Check sheet for the modelled part. Datum: model origin and axes. Units: mm. Face numbers are marked on the shaded views. A direction names the side the tool comes from. Coordinates: 2 decimals unless noted, no trailing zeros. Write each loop counter-clockwise with the first axis right and the second up, starting at its lowest first coordinate (ties: lowest second). Pieces come first, ordered by that corner, then holes. Notation, with made-up numbers: (84.5, 40.5) -> (114.5, 40.5) arc R22 cw to (114.5, 50.5) -> close; hole circle Ø1 at (-25.5, 51). An arc over 180 degrees is marked (long way). One line per item, written item: value. Start each with the question number.
1) Scan lines: line 1 along Y through (x, z) = (0, -3.25); line 2 along Y through (x, z) = (12, -1.5); line 3 along Z through (x, y) = (-11, -18.5). Record each from-to range of solid material in increasing order. Write a range as [from, to].
2) Set-up check for the marked faces 1, 2 and 3: record each of +Z, -Z, +X, -X, +Y, -Y from which the full face is reachable in a straight line by a thin tool's end or side.
3) Gauge pin test, flat ends, axial feed: P1, Ø1.6, axis at x = 12.5, y = 0, coming from the -Z side; P2, Ø3, axis at y = -8.5, z = 20.5, coming from the +X side (3 decimals); P3, Ø8, axis at y = -6.5, z = 30, coming from the -X side. Record the tip position at first contact, or that the pin passes through.
4) Sectioned sample at D-D on z = 18.5. Enter the section's corners in (x, y).
5) Sectioned sample at C-C on z = -1. Enter the section's corners in (x, y).
6) Sectioned sample at A-A on y = 0. Enter the section's corners in (x, z), plus the area to 3 significant figures.
```python
from build123d import *

# Parameters (mm, degrees)
SKETCH1_R           = 24
SKETCH1_R_2         = 1
BOSS_EXTRUDE1_DEPTH = 9.4
SKETCH1_4_R         = 20
SKETCH1_4_R_2       = 17.5
SKETCH1_4_R_3       = 1
BOSS_EXTRUDE2_DEPTH = 37
SKETCH1_5_R         = 17.5
SKETCH1_5_R_2       = 1
BOSS_EXTRUDE3_DEPTH = 4.5


with BuildPart() as part:
    # Sketch1 → Boss-Extrude1 (new body)
    with BuildSketch(Plane.XY):
        Circle(SKETCH1_R)
        with Locations((0, 12.5)):
            Circle(SKETCH1_R_2, mode=Mode.SUBTRACT)
        with Locations((12.5, 0)):
            Circle(SKETCH1_R_2, mode=Mode.SUBTRACT)
        with Locations((0, -12.5)):
            Circle(SKETCH1_R_2, mode=Mode.SUBTRACT)
        with Locations((-12.5, 0)):
            Circle(SKETCH1_R_2, mode=Mode.SUBTRACT)
    extrude(amount=BOSS_EXTRUDE1_DEPTH)

    # Sketch1_4 → Boss-Extrude2 (add)
    # profile 1 of 6: a face of its own
    with BuildSketch(Plane.XY):
        Circle(SKETCH1_4_R)
        Circle(SKETCH1_4_R_2, mode=Mode.SUBTRACT)
    # profile 2 of 6: a face of its own
    with BuildSketch(Plane.XY):
        Circle(SKETCH1_4_R_2)
        with Locations((-12.5, 0)):
            Circle(SKETCH1_4_R_3, mode=Mode.SUBTRACT)
        with Locations((0, -12.5)):
            Circle(SKETCH1_4_R_3, mode=Mode.SUBTRACT)
        with Locations((12.5, 0)):
            Circle(SKETCH1_4_R_3, mode=Mode.SUBTRACT)
        with Locations((0, 12.5)):
            Circle(SKETCH1_4_R_3, mode=Mode.SUBTRACT)
    # profile 3 of 6: a face of its own
    with BuildSketch(Plane.XY):
        with Locations((0, 12.5)):
            Circle(SKETCH1_4_R_3)
    # profile 4 of 6: a face of its own
    with BuildSketch(Plane.XY):
        with Locations((-12.5, 0)):
            Circle(SKETCH1_4_R_3)
    # profile 5 of 6: a face of its own
    with BuildSketch(Plane.XY):
        with Locations((12.5, 0)):
            Circle(SKETCH1_4_R_3)
    # profile 6 of 6: a face of its own
    with BuildSketch(Plane.XY):
        with Locations((0, -12.5)):
            Circle(SKETCH1_4_R_3)
    extrude(amount=BOSS_EXTRUDE2_DEPTH)

    # Sketch1_5 → Boss-Extrude3 (add)
    with BuildSketch(Plane.XY):
        Circle(SKETCH1_5_R)
        with Locations((0, 12.5)):
            Circle(SKETCH1_5_R_2, mode=Mode.SUBTRACT)
        with Locations((12.5, 0)):
            Circle(SKETCH1_5_R_2, mode=Mode.SUBTRACT)
        with Locations((0, -12.5)):
            Circle(SKETCH1_5_R_2, mode=Mode.SUBTRACT)
        with Locations((-12.5, 0)):
            Circle(SKETCH1_5_R_2, mode=Mode.SUBTRACT)
    extrude(amount=-BOSS_EXTRUDE3_DEPTH)


solid = part.part
```
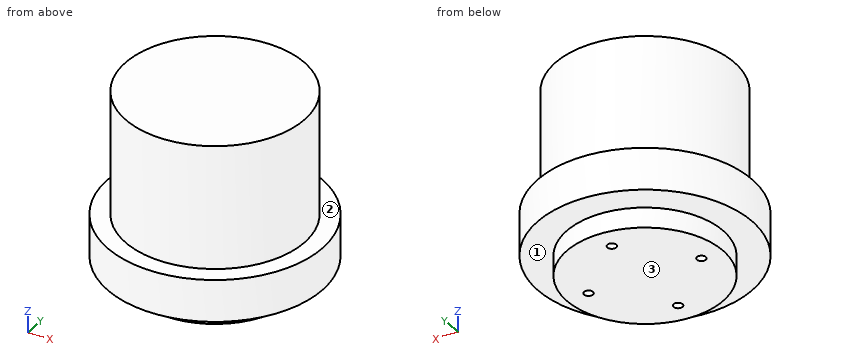
Answers:
1. line 1: y = [-17.5, -13.5], [-11.5, 11.5], [13.5, 17.5]
1. line 2: y = [-12.74, -0.87], [0.87, 12.74]
1. line 3: z = [0, 9.4]
2. face 1: -Z
2. face 2: +Z
2. face 3: -Z, +X, -X, +Y, -Y
3. P1: stops at z = 0
3. P2: stops at x = 18.735
3. P3: stops at x = -19.84
4. outline: circle Ø40 at (0, 0)
5. outline: circle Ø35 at (0, 0); hole circle Ø2 at (-12.5, 0); hole circle Ø2 at (0, -12.5); hole circle Ø2 at (0, 12.5); hole circle Ø2 at (12.5, 0)
6. outline: (-24, 0) -> (-17.5, 0) -> (-17.5, -4.5) -> (-13.5, -4.5) -> (-13.5, 0) -> (-11.5, 0) -> (-11.5, -4.5) -> (11.5, -4.5) -> (11.5, 0) -> (13.5, 0) -> (13.5, -4.5) -> (17.5, -4.5) -> (17.5, 0) -> (24, 0) -> (24, 9.4) -> (20, 9.4) -> (20, 37) -> (-20, 37) -> (-20, 9.4) -> (-24, 9.4) -> close
6. area: 1,690 mm2
